```python
from build123d import *

# Parameters (mm, degrees)
F0_W     = 254
F0_H     = 139.7
F1_DEPTH = 12.7
F2_R     = 22.156791
F2_R_2   = 22.69355
F2_R_3   = 59.134775
F2_W     = 33.248223
F2_H     = 78.026086
F3_DEPTH = 12.7


with BuildPart() as f1:
    # F0 (on Top) → F1 (new body)
    with BuildSketch(Plane.XY):
        with Locations((3.791939, -2.102413)):
            Rectangle(F0_W, F0_H)
    extrude(amount=F1_DEPTH)

    # F2 (on face) → F3 (join)
    with BuildSketch(Plane.XY.offset(12.7)):
        with Locations((-78.758061, 38.266217)):
            Circle(F2_R)
        with Locations((-78.758061, -30.959498)):
            Circle(F2_R_2)
        with Locations((12.287973, 0)):
            Circle(F2_R_3)
        with Locations((99.749218, 5.104106)):
            Rectangle(F2_W, F2_H)
    extrude(amount=F3_DEPTH)


solid = f1.part
```
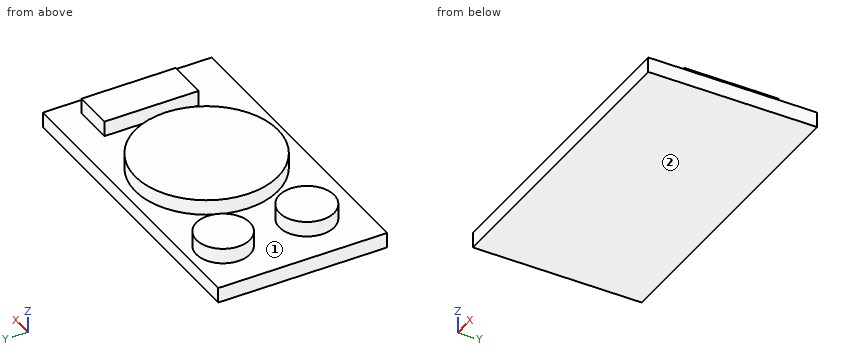
The listing builds one solid part. Answer for the finished solid, in the listing's coordinates (mm). Face numbers are marked on the shaded views. Coordinates: 2 decimals unless noted, no trailing zeros. Order: outer loops, then holes, each group sorted by start corner. A loop starts at its lowest first (then second) coordinate and runs counter-clockwise, first axis right, second up. Notation, with made-up numbers: M -11,-37 L 13,-37 A9 ccw 13,-20 Z; hole C 7.25,41 d6. An arc over 180 degrees is marked long. Answer as a JSON object with one key per item and string values. Group by question number.
1. Section B-B on y = 0 is taken. Write down the section's boundary in (x, z).
2. Flat-ended cylindrical pins translate along their axes: P1, Ø8, axis at x = -57.5, z = 18.5, coming from the -Y side; P2, Ø4, axis at y = -13, z = 19, coming from the +X side. Find the tip coordinate at first contact, or state that the pin passes through.
3. Section C-C on x = -36 is taken. Write down the section's boundary in (y, z), then the cut area to 3 significant figures.
4. Determine the mould class of the marked faces 1 and 2 for opening direction X: released by +X, released by -X, zero draft, split by the parting line, or undercut.
5. Section A-A on x = 96.5 is taken. Write down the section's boundary in (y, z), then the cut area to 3 significant figures.
6. Straight lines are drawn through the part: line 1 (X direction, y = 25.5, z = 21); line 2 (Z direction, x = -44.5, y = -23.5); line 3 (X direction, y = 21, z = 17.75). For each, find the intervals that lie inside material, in ascending order.
7. Section D-D on x = -69.5 is taken. Write down the section's boundary in (y, z), then the cut area to 3 significant figures.
Values follow:
{
 "1": {"outline": "M -123.21,0 L 130.79,0 L 130.79,12.7 L 116.37,12.7 L 116.37,25.4 L 83.13,25.4 L 83.13,12.7 L 71.42,12.7 L 71.42,25.4 L -46.85,25.4 L -46.85,12.7 L -123.21,12.7 Z"},
 "2": {"P1": "y = -45.7", "P2": "x = 116.37"},
 "3": {"outline": "M -71.95,0 L 67.75,0 L 67.75,12.7 L 34.13,12.7 L 34.13,25.4 L -34.13,25.4 L -34.13,12.7 L -71.95,12.7 Z", "area": "2,640 mm2"},
 "4": {"face 1": "undercut", "face 2": "zero draft"},
 "5": {"outline": "M -71.95,0 L 67.75,0 L 67.75,12.7 L 44.12,12.7 L 44.12,25.4 L -33.91,25.4 L -33.91,12.7 L -71.95,12.7 Z", "area": "2,770 mm2"},
 "6": {"line 1": "-96.87 to -60.65, -41.07 to 65.64, 83.13 to 116.37", "line 2": "0 to 12.7", "line 3": "-92.64 to -64.87, -42.99 to 67.57, 83.13 to 116.37"},
 "7": {"outline": "M -71.95,0 L 67.75,0 L 67.75,12.7 L 58.4,12.7 L 58.4,25.4 L 18.14,25.4 L 18.14,12.7 L -10.24,12.7 L -10.24,25.4 L -51.68,25.4 L -51.68,12.7 L -71.95,12.7 Z", "area": "2,810 mm2"}
}
